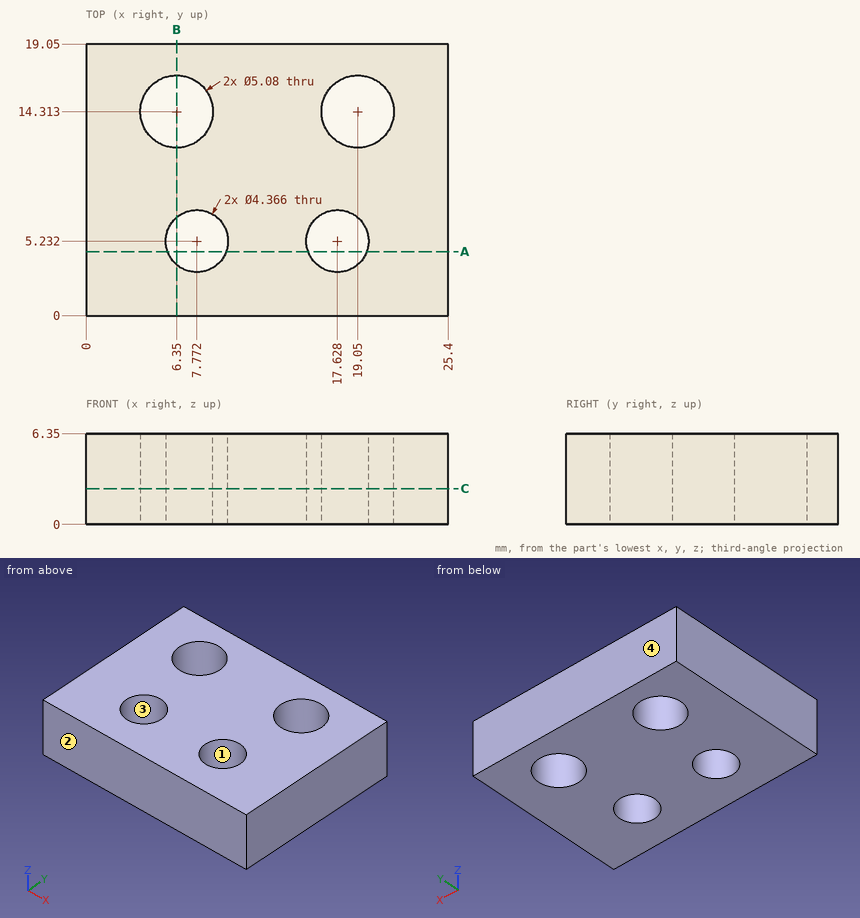
Could you check a few things on this drawing? It's one solid part, dimensions in mm from its lowest x, y, z. Coordinates: 2 decimals unless noted, no trailing zeros. Order: outer loops, then holes, each group sorted by start corner. A loop starts at its lowest first (then second) coordinate and runs counter-clockwise, first axis right, second up. Notation, with made-up numbers: (20, -26.5) - (42, -26.5) arc R24 cw to (42, -12.5) - close; hole circle Ø9 at (8, 29). An arc over 180 degrees is marked (long way). Answer as a JSON object with one key per item and string values. Group by question number.
Q1. Will this pin go through, and if not, where does the flat tip stop? P1, Ø6.5, axis at x = 19.05, y = 14.31, coming from the -Z side.
Q2. I need wall thicknesses on line 1 (X direction, y = 12.75, z = 0.75); line 2 (X direction, y = 15.25, z = 5.25); line 3 (Y direction, x = 7.5, z = 4). Which ranges of each line are inside material? Lowest first, please. Write a range as from..to.
Q3. Imagine slicing it at A-A (y = 4.5). Please give me the cut outline in (x, z), and give its area (3 significant figures).
Q4. We'd pull the mould along Y, two halves only. Please class the marked faces 1, 2, 3 and 4: +Y half, -Y half, draft (parallel to the pull), parting line (faces both ways), or undercut.
Q5. Imagine slicing it at B-B (x = 6.35). Please give me the cut outline in (y, z).
Q6. Imagine slicing it at C-C (z = 2.5). Give the number of separate pieces and of enclosed holes in the cut face.
Determined:
{
 "1": {"P1": "stops at z = 0"},
 "2": {"line 1": "x = 0..4.35, 8.35..17.05, 21.05..25.4", "line 2": "x = 0..3.99, 8.71..16.69, 21.41..25.4", "line 3": "y = 0..3.07, 7.4..12.05, 16.58..19.05"},
 "3": {"outline": "(0, 0) - (5.72, 0) - (5.72, 6.35) - (0, 6.35) - close; (9.83, 0) - (15.57, 0) - (15.57, 6.35) - (9.83, 6.35) - close; (19.68, 0) - (25.4, 0) - (25.4, 6.35) - (19.68, 6.35) - close", "area": "109 mm2"},
 "4": {"face 1": "undercut", "face 2": "-Y half", "face 3": "undercut", "face 4": "+Y half"},
 "5": {"outline": "(0, 0) - (3.58, 0) - (3.58, 6.35) - (0, 6.35) - close; (6.89, 0) - (11.77, 0) - (11.77, 6.35) - (6.89, 6.35) - close; (16.85, 0) - (19.05, 0) - (19.05, 6.35) - (16.85, 6.35) - close"},
 "6": {"separate pieces": "1", "enclosed holes": "4"}
}
